Input: part model. Units: mm. Frame: model coordinates. Face numbers are marked on the shaded views. A direction names the side the tool comes from. Give positions to 0.01 mm unless a question says otherwise; leave off trailing zeros. Write each loop counter-clockwise with the first axis right and the second up, starting at its lowest first coordinate (ties: lowest second). Pieces come first, ordered by that corner, then holes. Notation, with made-up numbers: (-22.5, 54) -> (2.5, 54) arc R16 ccw to (2.5, 58) -> close; hole circle Ø5 at (13, 70). An arc over 180 degrees is marked (long way). Answer as a JSON object with one key per item and string values. Group by question number.
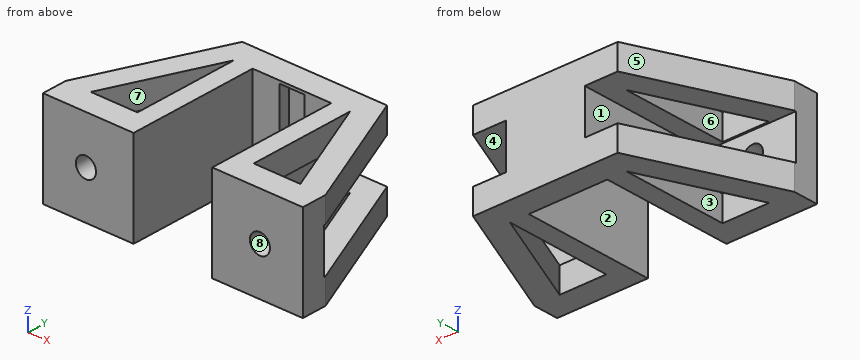
from build123d import *

# Parameters (mm, degrees)
PAD024_DEPTH       = 7.5
SKETCH062_W        = 16.391504
SKETCH062_H        = 7
POCKET003023_DEPTH = 22
SKETCH060_R        = 1.6
POCKET003024_DEPTH = 5.735743
SKETCH063_W        = 4
SKETCH063_H        = 12.856441
POCKET003025_DEPTH = 2


with BuildPart() as part:
    # Sketch061 → Pad024 (new body, symmetric)
    with BuildSketch(Plane.XY.offset(19.55)):
        Polygon((-11.506902, 93.265257), (11.506902, 93.265257), (20.658167, 72.265257), (20.658167, 68.265257), (6.25, 68.265257), (6.25, 89.265257), (-6.25, 89.265257), (-6.25, 68.265257), (-20.658167, 68.265257), (-20.658167, 72.265257), align=None)
        Polygon((-9.25, 72.265257), (-16.658167, 72.265257), (-9.25, 89.265257), align=None, mode=Mode.SUBTRACT)
        Polygon((9.25, 89.265257), (9.25, 72.265257), (16.658167, 72.265257), align=None, mode=Mode.SUBTRACT)
    extrude(amount=PAD024_DEPTH, both=True)

    # Sketch062 → Pocket003023 (cut)
    with BuildSketch(Plane.XZ.offset(-94)):
        with Locations((14.465183, 19.55)):
            Rectangle(SKETCH062_W, SKETCH062_H)
    pocket003023 = extrude(amount=POCKET003023_DEPTH, mode=Mode.SUBTRACT)

    # Mirrored003: Pocket003023 across Sketch062 V_Axis
    add(pocket003023.mirror(Plane(origin=(0, 94, 0), x_dir=(0, -1, 0), z_dir=(1, 0, 0))), mode=Mode.SUBTRACT)

    # Sketch060 → Pocket003024 (cut, through all)
    with BuildSketch(Plane.XZ.offset(-74)):
        with Locations((-13.83, 19.55)):
            Circle(SKETCH060_R)
        with Locations((13.83, 19.55)):
            Circle(SKETCH060_R)
    extrude(amount=POCKET003024_DEPTH, mode=Mode.SUBTRACT)

    # Sketch063 → Pocket003025 (cut)
    with BuildSketch(Plane.XZ.offset(-89)):
        with Locations((0, 20.182275)):
            Rectangle(SKETCH063_W, SKETCH063_H)
    extrude(amount=-POCKET003025_DEPTH, mode=Mode.SUBTRACT)


with BuildPart() as part_1:
    # Body012 placement: moved
    add(part.part.moved(Location((0, 2.5, 0))))


solid = part_1.part
1. Section D-D (z = 14.5). Return the cut outline in (x, y).
2. Mould query, pull axis Y, two halves, no side actions, for the marked faces 5, 6, 7 and 8. Classes: pulls with the +Y half, pulls with the -Y half, needs draft (parallel to the pull), parting line crosses it, or undercut.
3. Section A-A (z = 19.55). Return the cut outline in (x, y).
4. Section B-B (x = -13). Return the cut outline in (y, z), plus the area to 3 significant figures.
5. Line query: line 1 (X direction, y = 73, z = 19.55); line 2 (X direction, y = 88, z = 16); line 3 (Z direction, x = 11, y = 89). Output: solid intervals per line, ascending.
6. Reachability of the marked faces 1, 2, 3 and 4 from +Z, -Z, +X, -X, +Y, -Y: full face, straight path, thin tool, end or side. Return the list, or none.
7. Contact query for flat-ended pins moving along their axis: pin 1 Ø0.9 at (y, z) = (93, 22) entering from -X; pin 2 Ø3 at (y, z) = (86, 13.5) entering from +X; pin 3 Ø4.5 at (y, z) = (82, 23) entering from -X. Output: stop coordinate, or through.
8. Section C-C (y = 82.25). State how many separate pieces and enclosed holes the cut face has, plus the area to 3 significant figures.
Working result:
{
 "1": {"outline": "(-20.66, 70.77) -> (-6.25, 70.77) -> (-6.25, 91.77) -> (-2, 91.77) -> (-2, 93.5) -> (2, 93.5) -> (2, 91.77) -> (6.25, 91.77) -> (6.25, 70.77) -> (20.66, 70.77) -> (20.66, 74.77) -> (11.51, 95.77) -> (-11.51, 95.77) -> (-20.66, 74.77) -> close; hole (-16.66, 74.77) -> (-9.25, 74.77) -> (-9.25, 91.77) -> close; hole (9.25, 74.77) -> (16.66, 74.77) -> (9.25, 91.77) -> close"},
 "2": {"face 5": "pulls with the +Y half", "face 6": "undercut", "face 7": "undercut", "face 8": "needs draft"},
 "3": {"outline": "(-20.66, 70.77) -> (-15.43, 70.77) -> (-15.43, 74.5) -> (-20.66, 74.5) -> close; (-12.23, 70.77) -> (-6.25, 70.77) -> (-6.25, 91.77) -> (-2, 91.77) -> (-2, 93.5) -> (2, 93.5) -> (2, 91.77) -> (6.25, 91.77) -> (6.25, 70.77) -> (12.23, 70.77) -> (12.23, 74.5) -> (6.27, 74.5) -> (6.27, 95.77) -> (-6.27, 95.77) -> (-6.27, 74.5) -> (-12.23, 74.5) -> close; (15.43, 70.77) -> (20.66, 70.77) -> (20.66, 74.5) -> (15.43, 74.5) -> close"},
 "4": {"outline": "(70.77, 12.05) -> (74.77, 12.05) -> (74.77, 16.05) -> (74.5, 16.05) -> (74.5, 18.18) -> (70.77, 18.18) -> close; (70.77, 20.92) -> (74.5, 20.92) -> (74.5, 23.05) -> (74.77, 23.05) -> (74.77, 27.05) -> (70.77, 27.05) -> close; (83.16, 12.05) -> (92.34, 12.05) -> (92.34, 16.05) -> (83.16, 16.05) -> close; (83.16, 23.05) -> (92.34, 23.05) -> (92.34, 27.05) -> (83.16, 27.05) -> close", "area": "121 mm^2"},
 "5": {"line 1": "x = -20.66 to -15.43, -12.23 to -6.25, 6.25 to 12.23, 15.43 to 20.66", "line 2": "x = -14.89 to -10.89, -9.25 to -6.25, 6.25 to 9.25, 10.89 to 14.89", "line 3": "z = 12.05 to 16.05, 23.05 to 27.05"},
 "6": {"face 1": "-X, +Y", "face 2": "+Z, -Z, -Y", "face 3": "+Z, -Z", "face 4": "+X, +Y"},
 "7": {"pin 1": "stops at x = -6.27", "pin 2": "stops at x = 16.42", "pin 3": "stops at x = -18.49"},
 "8": {"separate pieces": "6", "enclosed holes": "0", "area": "112 mm^2"}
}
